Verification items for the finished model (mm, model axes). Face numbers are marked on the shaded views. Coordinates: 2 decimals unless noted, no trailing zeros. Write each loop counter-clockwise with the first axis right and the second up, starting at its lowest first coordinate (ties: lowest second). Pieces come first, ordered by that corner, then holes. Notation, with made-up numbers: (57, 33.5) -> (96, 33.5) arc R3 ccw to (96, 38.5) -> close; hole circle Ø3 at (-24.75, -6). An arc over 180 degrees is marked (long way). Answer in a Markdown table with one row per item.
```python
from build123d import *

# Parameters (mm, degrees)
F3_DEPTH = 30


with BuildPart() as f1:
    # F0 (on Front) → F1 (revolve)
    with BuildSketch(Plane.XZ):
        Polygon((-3.454545, -17.869791), (-3.454545, -20.869791), (-0.454545, -20.869791), (4.545455, -20.869791), (4.545455, 5.130209), (-0.454545, 5.130209), (-0.454545, -10.198509), (-1.454545, -15.869791), align=None)
    revolve(axis=Axis((4.545455, 0, -7.869791), (0, 0, -1)))

    # F2 (on face) → F3 (cut)
    with BuildSketch(Plane(origin=(0, 0, -20.869791), x_dir=(1, 0, 0), z_dir=(0, 0, -1))):
        with BuildLine():
            Line((5.640719, -4.498865), (5.640719, -3.847128))
            ThreePointArc((5.640719, -3.847128), (4.447064, 3.99879), (3.640719, -3.896339))
            Line((3.640719, -3.896339), (3.640719, -4.498865))
            Line((3.640719, -4.498865), (5.640719, -4.498865))
        make_face()
    extrude(amount=-F3_DEPTH, mode=Mode.SUBTRACT)


solid = f1.part
```
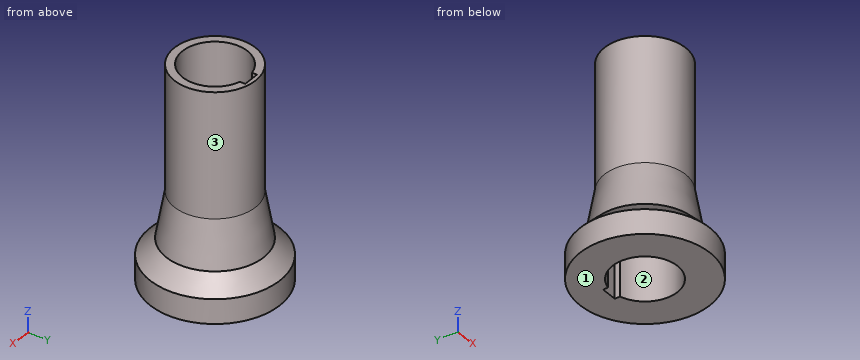
1. Sectioned sample at B-B, the plane z = -2.5. Record the cut outline in (x, y), and give its area (3 significant figures).
Findings below:
| item | result |
|---|---|
| outline | circle Ø10 at (4.55, 0); hole (3.64, 3.9) arc R4 ccw (long way) to (5.64, 3.85) -> (5.64, 4.5) -> (3.64, 4.5) -> close |
| area | 27.2 mm² |
2. Go/stop test with flat-tipped pins: pin 1 (3 mm diameter, centred on x = 6, z = -17, fed in from +Y); pin 2 (5 mm diameter, centred on x = 3.5, z = -10.5, fed in from -Y); pin 3 (0.7 mm diameter, centred on y = 4.5, z = -13.5, fed in from +X). Record where each tip stops, or that it passes through.
Findings below:
| item | result |
|---|---|
| pin 1 | stops at y = 8 |
| pin 2 | stops at y = -5.47 |
| pin 3 | stops at x = 8.29 |
3. Sectioned sample at C-C, the plane z = -16.5. Record the cut outline in (x, y), and give its area (3 significant figures).
Findings below:
| item | result |
|---|---|
| outline | circle Ø13.26 at (4.55, 0); hole (3.64, 3.9) arc R4 ccw (long way) to (5.64, 3.85) -> (5.64, 4.5) -> (3.64, 4.5) -> close |
| area | 86.8 mm² |
4. Material ranges on probe 1 along X at (y, z) = (2, -4.5); probe 2 along X at (y, z) = (4, -2.5); probe 3 along Y at (x, z) = (2.5, -7.25), recorded low to high. Write a range as from..to.
Findings below:
| item | result |
|---|---|
| probe 1 | x = -0.04..1.08, 8.01..9.13 |
| probe 2 | x = 1.55..3.64, 5.64..7.55 |
| probe 3 | y = -4.56..-3.44, 3.44..4.56 |
5. Sectioned sample at A-A, the plane y = 0. Record the cut outline in (x, z).
Findings below:
| item | result |
|---|---|
| outline | (-3.45, -20.87) -> (0.55, -20.87) -> (0.55, 5.13) -> (-0.45, 5.13) -> (-0.45, -10.2) -> (-1.45, -15.87) -> (-3.45, -17.87) -> close; (8.55, -20.87) -> (12.55, -20.87) -> (12.55, -17.87) -> (10.55, -15.87) -> (9.55, -10.2) -> (9.55, 5.13) -> (8.55, 5.13) -> close |
6. Release check for a two-part mould opening along Y. For the marked faces 1, 2 and 3 record: released by +Y, released by -Y, zero draft, split by the parting line, or undercut.
Findings below:
| item | result |
|---|---|
| face 1 | zero draft |
| face 2 | undercut |
| face 3 | split by the parting line |
